```python
from build123d import *

# Parameters (mm, degrees)
F1_DEPTH = 50
F2_R     = 5


with BuildPart() as f1:
    # F0 (on Front) → F1 (new body, symmetric)
    with BuildSketch(Plane.XZ):
        with BuildLine():
            Line((15.126235, 37.558659), (15.126235, -39.941341))
            Line((15.126235, -39.941341), (19.126235, -39.941341))
            Line((19.126235, -39.941341), (19.126235, 42.558659))
            ThreePointArc((19.126235, 42.558659), (18.394002, 44.326426), (16.626235, 45.058659))
            Line((16.626235, 45.058659), (0.126235, 45.058659))
            Line((0.126235, 45.058659), (-16.373765, 45.058659))
            ThreePointArc((-16.373765, 45.058659), (-18.141532, 44.326426), (-18.873765, 42.558659))
            Line((-18.873765, 42.558659), (-18.873765, -39.941341))
            Line((-18.873765, -39.941341), (-14.873765, -39.941341))
            Line((-14.873765, -39.941341), (-14.873765, 37.558659))
            ThreePointArc((-14.873765, 37.558659), (-14.141532, 39.326426), (-12.373765, 40.058659))
            Line((-12.373765, 40.058659), (12.626235, 40.058659))
            ThreePointArc((12.626235, 40.058659), (14.394002, 39.326426), (15.126235, 37.558659))
        make_face()
    extrude(amount=F1_DEPTH, both=True)

    # F2
    f2_edges = [f1.edges().sort_by_distance(p)[0] for p in [
        (17.126235, -50, -39.941341),
        (-16.873765, -50, -39.941341),
        (17.126235, 50, -39.941341),
        (-16.873765, 50, -39.941341),
    ]]
    fillet(f2_edges, radius=F2_R)


solid = f1.part
```
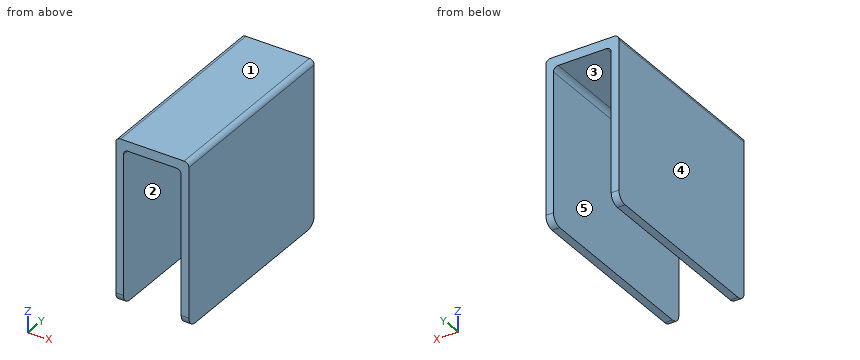
The model under review builds one solid part; all positions refer to its coordinate system, in mm. Face numbers are marked on the shaded views. A direction names the side the tool comes from. Round coordinates to 2 decimals unless told otherwise and drop trailing zeros. Loops run counter-clockwise (first coordinate to the right, second up) from the corner with the lowest first, then second, coordinate; pieces in that order, holes last. Notation, with made-up numbers: (-33.5, 11.5) -> (8.5, 11.5) arc R30 cw to (8.5, 42.5) -> close; hole circle Ø4 at (-3.5, 21). An arc over 180 degrees is marked (long way). Answer as a JSON object with one key per item and string values. Group by question number.
1) Mouldability with a two-part tool opening along Z and no side actions: class the marked faces 1, 2 and 3 as released by +Z, released by -Z, zero draft, split by the parting line, or undercut.
2) We need section C-C on x = -6. Write out the cut boundary in (y, z), then the cut area to 3 significant figures.
3) We need section A-A on z = -32. Write out the cut boundary in (x, y), then the cut area to 3 significant figures.
4) For line 1 (X direction, y = -34.5, z = -2); line 2 (Z direction, x = 3.5, y = 16); line 3 (Z direction, x = -17, y = -17), list the stretches that pass through material, from the lowest coordinate up. Write a range as [from, to].
5) For pin 1 Ø20 at (x, y) = (2.5, 3) entering from -Z; pin 2 Ø10 at (x, z) = (-7.5, -11.5) entering from +Y; pin 3 Ø3 at (x, z) = (14, 31) entering from -Y, all flat-tipped, find the tip position at first contact; note any pin that passes through.
6) For the marked faces 4 and 5, list the 3-axis set-ups (+Z, -Z, +X, -X, +Y, -Y) from which the entire face can be reached by the end or side of a thin tool; tool diameter is ignored.
7) We need section B-B on y = -28.5. Write out the cut boundary in (x, z).
Result set:
{
 "1": {"face 1": "released by +Z", "face 2": "zero draft", "face 3": "released by -Z"},
 "2": {"outline": "(-50, 40.06) -> (50, 40.06) -> (50, 45.06) -> (-50, 45.06) -> close", "area": "500 mm²"},
 "3": {"outline": "(-18.87, -50) -> (-14.87, -50) -> (-14.87, 50) -> (-18.87, 50) -> close; (15.13, -50) -> (19.13, -50) -> (19.13, 50) -> (15.13, 50) -> close", "area": "800 mm²"},
 "4": {"line 1": "[-18.87, -14.87], [15.13, 19.13]", "line 2": "[40.06, 45.06]", "line 3": "[-39.94, 44.98]"},
 "5": {"pin 1": "z = 40.06", "pin 2": "through", "pin 3": "y = -50"},
 "6": {"face 4": "+Z, -Z, -X, +Y, -Y", "face 5": "-Z, +Y, -Y"},
 "7": {"outline": "(-18.87, -39.94) -> (-14.87, -39.94) -> (-14.87, 37.56) arc R2.5 cw to (-12.37, 40.06) -> (12.63, 40.06) arc R2.5 cw to (15.13, 37.56) -> (15.13, -39.94) -> (19.13, -39.94) -> (19.13, 42.56) arc R2.5 ccw to (16.63, 45.06) -> (-16.37, 45.06) arc R2.5 ccw to (-18.87, 42.56) -> close"}
}
